Geometry: final body of the model. Coordinates: model frame, mm. Coordinates: 2 decimals unless noted, no trailing zeros. Order: outer loops, then holes, each group sorted by start corner. A loop starts at its lowest first (then second) coordinate and runs counter-clockwise, first axis right, second up. Notation, with made-up numbers: M 36.25,71.25 L 55.25,71.25 A27 cw 55.25,103.25 Z; hole C 76.25,26.5 d4. An arc over 180 degrees is marked long. Use CSV: the item, a comma, the result in double quotes. Start each with the question number.
1. Material intervals for line 1 (Y direction, x = 76, z = -2.15); line 2 (Y direction, x = -57, z = -4) (3 decimals); line 3 (X direction, y = -4.5, z = -1.65) (3 decimals), sorted ascending.
2. Section query B-B on z = -1.8. State how many separate pieces and enclosed holes the cut face has, and give its area (3 significant figures).
3. Section query A-A on x = -36. Return the cut outline in (y, z).
4. Pull-direction query (X, two-part tool) for faces 1 (the flat face through (21, 0, 0)), 2 (the flat face through (-70.348, 19.577, -2.354)), 3 (the flat face through (63.5, -18, -2)); classes: pulls with the +X half, pulls with the -X half, needs draft (parallel to the pull), parting line crosses it, or undercut.
from build123d import *

# Parameters (mm, degrees)
SKETCH1_R          = 1.3890625
SKETCH1_R_2        = 1.984375
EXTRUDE1_DEPTH     = 4.7752
SKETCH9_R          = 1.4732
SKETCH9_R_2        = 1.984375
CUT_EXTRUDE3_DEPTH = 4.7752


with BuildPart() as part:
    # Sketch1 → Extrude1 (new body)
    with BuildSketch(Plane.XY):
        with BuildLine():
            Line((-23.0124, 30.1498), (111.125, 30.1498))
            Line((111.125, 30.1498), (111.125, -30.1498))
            Line((111.125, -30.1498), (-23.0124, -30.1498))
            Line((-23.0124, -30.1498), (-116.376349272, -9.295934526))
            ThreePointArc((-116.376349272, -9.295934526), (-123.825, 0), (-116.376349272, 9.295934526))
            Line((-116.376349272, 9.295934526), (-23.0124, 30.1498))
        make_face()
        with Locations((-114.3, 0)):
            Circle(SKETCH1_R, mode=Mode.SUBTRACT)
        with Locations((104.775, -20.5105)):
            Circle(SKETCH1_R_2, mode=Mode.SUBTRACT)
        with Locations((92.075, -20.5105)):
            Circle(SKETCH1_R_2, mode=Mode.SUBTRACT)
        with Locations((104.775, 20.5105)):
            Circle(SKETCH1_R_2, mode=Mode.SUBTRACT)
        with Locations((92.075, 20.5105)):
            Circle(SKETCH1_R_2, mode=Mode.SUBTRACT)
        with BuildLine():
            Line((-93.787006647, 9.448644842), (-43.351349272, 20.714003926))
            ThreePointArc((-43.351349272, 20.714003926), (-35.318977914, 18.85119969), (-31.75, 11.4180694))
            Line((-31.75, 11.4180694), (-31.75, 9.525))
            ThreePointArc((-31.75, 9.525), (-33.609871939, 5.034871939), (-38.1, 3.175))
            Line((-38.1, 3.175), (-93.094890223, 3.175))
            ThreePointArc((-93.094890223, 3.175), (-96.250743703, 6.001842258), (-93.787006647, 9.448644842))
        make_face(mode=Mode.SUBTRACT)
        with BuildLine():
            Line((-93.787006647, -9.448644842), (-43.351349272, -20.714003926))
            ThreePointArc((-43.351349272, -20.714003926), (-35.318977914, -18.85119969), (-31.75, -11.4180694))
            Line((-31.75, -11.4180694), (-31.75, -9.525))
            ThreePointArc((-31.75, -9.525), (-33.609871939, -5.034871939), (-38.1, -3.175))
            Line((-38.1, -3.175), (-93.094890223, -3.175))
            ThreePointArc((-93.094890223, -3.175), (-96.250743703, -6.001842258), (-93.787006647, -9.448644842))
        make_face(mode=Mode.SUBTRACT)
        with BuildLine():
            Line((85.725, -23.7998), (85.725, -12.573))
            ThreePointArc((85.725, -12.573), (84.79506403, -10.32793597), (82.55, -9.398))
            Line((82.55, -9.398), (66.675, -9.398))
            ThreePointArc((66.675, -9.398), (64.42993597, -10.32793597), (63.5, -12.573))
            Line((63.5, -12.573), (63.5, -23.7998))
            ThreePointArc((63.5, -23.7998), (64.42993597, -26.04486403), (66.675, -26.9748))
            Line((66.675, -26.9748), (82.55, -26.9748))
            ThreePointArc((82.55, -26.9748), (84.79506403, -26.04486403), (85.725, -23.7998))
        make_face(mode=Mode.SUBTRACT)
        with BuildLine():
            Line((85.725, 23.7998), (85.725, 12.573))
            ThreePointArc((85.725, 12.573), (84.79506403, 10.32793597), (82.55, 9.398))
            Line((82.55, 9.398), (66.675, 9.398))
            ThreePointArc((66.675, 9.398), (64.42993597, 10.32793597), (63.5, 12.573))
            Line((63.5, 12.573), (63.5, 23.7998))
            ThreePointArc((63.5, 23.7998), (64.42993597, 26.04486403), (66.675, 26.9748))
            Line((66.675, 26.9748), (82.55, 26.9748))
            ThreePointArc((82.55, 26.9748), (84.79506403, 26.04486403), (85.725, 23.7998))
        make_face(mode=Mode.SUBTRACT)
    extrude(amount=-EXTRUDE1_DEPTH)

    # Sketch9 → Cut-Extrude3 (cut)
    with BuildSketch(Plane.XY):
        with Locations((-26.9875, 7.9248)):
            Circle(SKETCH9_R)
        with Locations((-9.525, -7.9248)):
            Circle(SKETCH9_R)
        with Locations((-26.9875, -7.9248)):
            Circle(SKETCH9_R)
        with Locations((11.90625, -26.9875)):
            Circle(SKETCH9_R_2)
        with Locations((-9.525, 7.9248)):
            Circle(SKETCH9_R)
        with Locations((11.90625, 26.9875)):
            Circle(SKETCH9_R_2)
        with Locations((30.95625, 0)):
            Circle(SKETCH9_R_2)
        with Locations((3.96875, -18.25625)):
            Circle(SKETCH9_R_2)
        with Locations((37.30625, -18.25625)):
            Circle(SKETCH9_R_2)
    extrude(amount=-CUT_EXTRUDE3_DEPTH, mode=Mode.SUBTRACT)


solid = part.part
Results list:
1,line 1,"y = -30.15 to -26.97, -9.4 to 9.4, 26.97 to 30.15"
1,line 2,"y = -22.558 to -17.665, -3.175 to 3.175, 17.665 to 22.558"
1,line 3,"x = -122.695 to -95.675, -34.218 to 111.125"
2,separate pieces,"1"
2,enclosed holes,"18"
2,area,"9,390 mm²"
3,outline,"M -27.25,-4.78 L -19.35,-4.78 L -19.35,0 L -27.25,0 Z; M -3.53,-4.78 L 3.53,-4.78 L 3.53,0 L -3.53,0 Z; M 19.35,-4.78 L 27.25,-4.78 L 27.25,0 L 19.35,0 Z"
4,face 1,"needs draft"
4,face 2,"pulls with the -X half"
4,face 3,"undercut"
